Check sheet for the modelled part. Datum: model origin and axes. Units: mm. Round coordinates to 2 decimals unless told otherwise and drop trailing zeros. Order: outer loops, then holes, each group sorted by start corner. A loop starts at its lowest first (then second) coordinate and runs counter-clockwise, first axis right, second up. Notation, with made-up numbers: M 62.5,-2.5 L 97.5,-2.5 A18 ccw 97.5,28.5 Z; hole C 14.5,59 d4. An arc over 180 degrees is marked long. One line per item, written item: value. Start each with the question number.
(1) Cross-section at D-D, the plane x = 40. Enter the section's corners in (y, z).
(2) Depth check by flat-ended pin: pin 1 Ø3 at (x, y) = (40.5, 7) entering from -Z; pin 2 Ø0.5 at (x, z) = (28.5, 0.5) entering from +Y. Enter the tip coordinate at first touch or a pass-through.
(3) Cross-section at C-C, the plane y = 4. Enter the section's corners in (x, z).
(4) Release check for a two-part mould opening along X. For faces 1 (the face through (73.28, 4.61, 0.3)), 2 (the face through (37, 4, 1)) record: released by +X, released by -X, zero draft, split by the parting line, or undercut.
(5) Cross-section at B-B, the plane z = 0.85. Enter the section's corners in (x, y), and give its area (3 significant figures).
(6) Cross-section at A-A, the plane x = 71.8. Enter the section's corners in (y, z), and give its area (3 significant figures).
(7) Thickness scan on L1, parallel to X at y = 6.25, z = 0.8; L2, parallel to Y at x = 3.2, z = 0.2; L3, parallel to Y at x = 35.5, z = 0.3. Record the ranges inside material, lowest first.
Autodesk Inventor part; units mm, degrees
ref_plane "YZ Plane" through (0, 0, 0) normal (1, 0, 0) x (0, 1, 0)
ref_plane "XZ Plane" through (0, 0, 0) normal (0, 1, 0) x (-1, 0, 0)
ref_plane "XY Plane" through (0, 0, 0) normal (0, 0, 1) x (1, 0, 0)
sketch "Sketch1" plane through (0, 0, 0) normal (0, 0, 1) x (1, 0, 0)
  line L0 (0, 0) -> (75, 0)
  line L1 (75, 0) -> (75, 10)
  line L2 (75, 10) -> (0, 10)
  line L3 (0, 10) -> (0, 0)
  line L4 (15, 10) -> (15, 5)
  line L5 (15, 5) -> (60, 5)
  line L6 (60, 5) -> (60, 10)
  circle A0 centre (3.2, 4) radius 1.6
  line L7 (37.5, 10) -> (37.5, 6.6559) construction
  circle A1 centre (71.8, 4) radius 1.6
  point P0 (0, 5)
  dimension "d0" = 75
  dimension "d1" = 10
  dimension "d3" = 5
  dimension "d4" = 45
  dimension "d5" = 3.2
  dimension "d7" = 4
  dimension "d10" = 3.2
extrude "Extrusion1" add sketch "Sketch1" along normal blind 1 contours L3 L2 L4 L5 L6 L1 L0
chamfer "Chamfer1" distance 0.4 angle 45 2 edges at (1.6, 4, 1) (70.2, 4, 1)
properties part number "oslonka"
Values found:
1. outline: M 0,0 L 5,0 L 5,1 L 0,1 Z
2. pin 1: through
2. pin 2: y = 5
3. outline: M 0,0 L 1.6,0 L 1.6,0.6 L 1.2,1 L 0,1 Z; M 4.8,0 L 70.2,0 L 70.2,0.6 L 69.8,1 L 5.2,1 L 4.8,0.6 Z; M 73.4,0 L 75,0 L 75,1 L 73.8,1 L 73.4,0.6 Z
4. face 1: undercut
4. face 2: zero draft
5. outline: M 0,0 L 75,0 L 75,10 L 60,10 L 60,5 L 15,5 L 15,10 L 0,10 Z; hole C 3.2,4 d3.7; hole C 71.8,4 d3.7
5. area: 503 mm^2
6. outline: M 0,0 L 2.4,0 L 2.4,0.6 L 2,1 L 0,1 Z; M 5.6,0 L 10,0 L 10,1 L 6,1 L 5.6,0.6 Z
6. area: 6.64 mm^2
7. L1: 0 to 15, 60 to 75
7. L2: 0 to 2.4, 5.6 to 10
7. L3: 0 to 5
